Answer from the drawing. Dimensions are ordinates in mm from the lowest x, y and z of the part. Give positions to 0.01 mm unless a question says otherwise; leave off trailing zeros. Loops run counter-clockwise (first coordinate to the right, second up) from the corner with the lowest first, then second, coordinate; pieces in that order, holes last. Notation, with made-up numbers: (34.25, 75.25) - (53.25, 75.25) arc R13 ccw to (53.25, 97.25) - close; hole circle Ø7 at (42, -12.5). An arc over 180 degrees is marked (long way). One line per question, with ' | ' between items. Start each with the question number.
1. Section B-B (y = 13.75) is taken. Determine the outline of the cut face in (x, z) (1 decimal).
2. For a pull along Y with two mould halves and no side action, classify the marked faces 1, 2, 3 and 4 as released by +Y, released by -Y, zero draft, split by the parting line, or undercut.
3. Section C-C (z = 4.4) is taken. Give the number of separate pieces and of enclosed holes in the cut face, plus the area to 3 significant figures.
4. Find the intervals of material crossed by line 1 (Y direction, x = 7, z = 2.6) (1 decimal); line 2 (Y direction, x = 18.5, z = 2.2) (1 decimal), in increasing order.
5. Section D-D (x = 24.5) is taken. Determine the outline of the cut face in (y, z) (1 decimal).
6. Section A-A (x = 30.5) is taken. Determine the outline of the cut face in (y, z) (1 decimal).
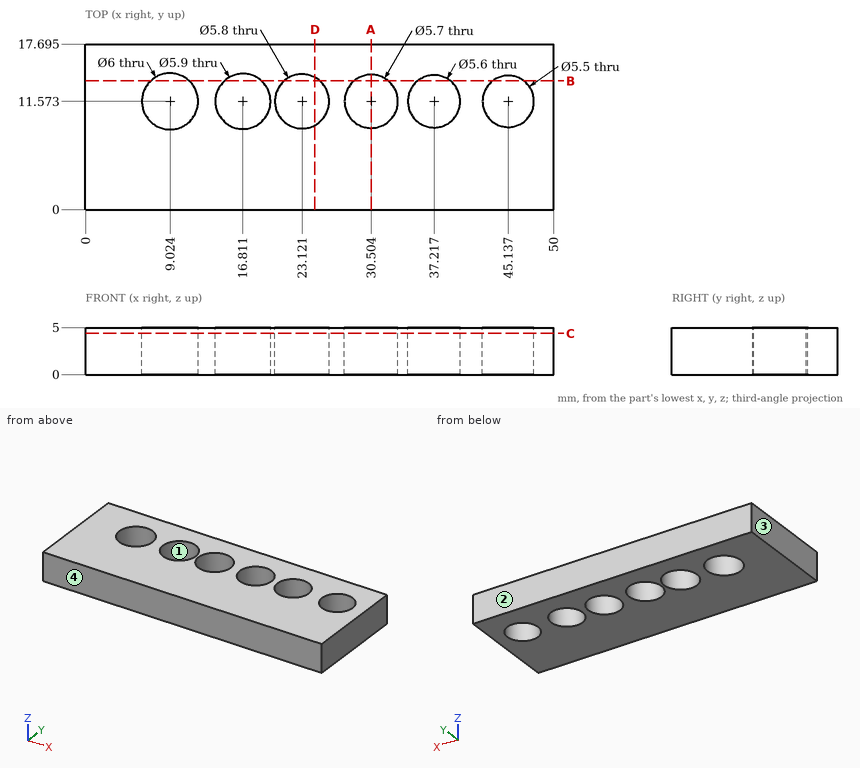
Conclusion:
1) outline: (0, 0) - (7, 0) - (7, 5) - (0, 5) - close; (11.1, 0) - (14.8, 0) - (14.8, 5) - (11.1, 5) - close; (18.8, 0) - (21.2, 0) - (21.2, 5) - (18.8, 5) - close; (25, 0) - (28.7, 0) - (28.7, 5) - (25, 5) - close; (32.3, 0) - (35.5, 0) - (35.5, 5) - (32.3, 5) - close; (39, 0) - (43.5, 0) - (43.5, 5) - (39, 5) - close; (46.8, 0) - (50, 0) - (50, 5) - (46.8, 5) - close
2) face 1: undercut | face 2: released by +Y | face 3: zero draft | face 4: released by -Y
3) separate pieces: 1 | enclosed holes: 6 | area: 729 mm²
4) line 1: 0 to 9.4, 13.8 to 17.7 | line 2: 0 to 9.2, 14 to 17.7
5) outline: (0, 0) - (9, 0) - (9, 5) - (0, 5) - close; (14.1, 0) - (17.7, 0) - (17.7, 5) - (14.1, 5) - close
6) outline: (0, 0) - (8.7, 0) - (8.7, 5) - (0, 5) - close; (14.4, 0) - (17.7, 0) - (17.7, 5) - (14.4, 5) - close
